from build123d import *

# Parameters (mm, degrees)
F4_W     = 4.316755
F4_H     = 4.316762
F5_DEPTH = 203.2


with BuildPart() as f3:
    # F0 (on Top) → F3 section 0
    with BuildSketch(Plane.XY, mode=Mode.PRIVATE) as f3_s0:
        Polygon((102.593086, 100.59711), (-100.59711, 102.593086), (-102.593086, -100.59711), (100.59711, -102.593086), align=None)
    loft([f3_s0.sketch, Vertex(0, 0, 152.4)])

    # F4 (on offset) → F5 (cut)
    with BuildSketch(Plane.XY.offset(152.4)):
        Polygon((0, 111.647069), (0, 0), (118.514635, 0), (118.514635, 107.330307), (114.19788, 107.330307), (114.19788, 111.647069), align=None)
        with Locations((116.356257, 109.488688)):
            Rectangle(F4_W, F4_H)
    extrude(amount=-F5_DEPTH, mode=Mode.SUBTRACT)


solid = f3.part
Here's how the part is built. I have some questions about the finished solid (model axes, mm). A direction names the side the tool comes from. Give positions to 0.01 mm unless a question says otherwise; leave off trailing zeros. Order: outer loops, then holes, each group sorted by start corner. A loop starts at its lowest first (then second) coordinate and runs counter-clockwise, first axis right, second up. Notation, with made-up numbers: (-32, 82.25) -> (-1, 82.25) arc R12 cw to (-1, 88.25) -> close; hole circle Ø4 at (83.25, 79.5). An arc over 180 degrees is marked (long way). Use a Markdown table: item, result. Add a question column.
Item 1: Imagine slicing it at D-D on z = 44.5. Please give me the cut outline in (x, y).
Item 2: For faces 1 (the face through (-26, -22, 0)), 2 (the face through (28, 0, 43)), which set-ups out of +Z, -Z, +X, -X, +Y, -Y let a thin tool reach every point of the face, with its end or its side?
Item 3: Imagine slicing it at C-C on y = -50. Please give me the cut outline in (x, z).
Item 4: Imagine slicing it at B-B on x = 86. Please give me the cut outline in (y, z).
Item 5: Will these pins go through, and if not, where does the flat tip stop? pin 1 (1.5 mm diameter, centred on y = -52.5, z = 44.5, fed in from +X); pin 2 (1 mm diameter, centred on x = 5, y = -73.5, fed in from +Z); pin 3 (3 mm diameter, centred on y = 16, z = 104.5, fed in from +X).
Item 6: Imagine slicing it at A-A on z = 16. Please give me the cut outline in (x, y), plus the area to 3 significant figures.
Item 7: I need wall thicknesses on line 1 (Z direction, x = -49, y = 6.5); line 2 (Y direction, x = -9.5, z = 36.5); line 3 (Z direction, x = -0.5, y = -7). Which ranges of each line are inside material? Lowest first, please.
Data:
| question | item | result |
|---|---|---|
| 1 | outline | (-72.64, -71.22) -> (71.22, -72.64) -> (71.94, 0) -> (0, 0) -> (0, 71.94) -> (-71.22, 72.64) -> close |
| 2 | face 1 | -Z, +X, -X, +Y, -Y |
| 2 | face 2 | +Z, -Z, +X, +Y |
| 3 | outline | (-102.1, 0) -> (101.11, 0) -> (49.03, 78.13) -> (-50.99, 76.65) -> close |
| 4 | outline | (-102.45, 0) -> (0, 0) -> (0, 23.41) -> (-87.71, 22.11) -> close |
| 5 | pin 1 | stops at x = 71.92 |
| 5 | pin 2 | stops at z = 42.98 |
| 5 | pin 3 | stops at x = 0 |
| 6 | outline | (-91.82, -90.04) -> (90.04, -91.82) -> (90.94, 0) -> (0, 0) -> (0, 90.94) -> (-90.04, 91.82) -> close |
| 6 | area | 24,800 mm² |
| 7 | line 1 | z = 0 to 78.81 |
| 7 | line 2 | y = -77.18 to 77.36 |
| 7 | line 3 | z = 0 to 141.89 |
